Geometry check sheet. Reference: the model listing, model coordinates, mm. A direction names the side the tool comes from. Round coordinates to 2 decimals unless told otherwise and drop trailing zeros. Write each loop counter-clockwise with the first axis right and the second up, starting at its lowest first coordinate (ties: lowest second). Pieces come first, ordered by that corner, then holes.
from build123d import *

# Parameters (mm, degrees)
BOSS_EXTRUDE1_DEPTH = 15.3
SHELL1_T            = 3
SKETCH2_W           = 7
SKETCH2_H           = 15.5
SKETCH2_W_2         = 3
SKETCH2_W_3         = 15.5
SKETCH2_H_2         = 7
SKETCH2_H_3         = 3
CUT_EXTRUDE1_DEPTH  = 5


with BuildPart() as part:
    # Sketch1 → Boss-Extrude1 (new body)
    with BuildSketch(Plane.XY):
        Polygon((0, 0), (15.5, 0), (15.5, 30), (45.5, 30), (45.5, 45.5), (0, 45.5), align=None)
    extrude(amount=BOSS_EXTRUDE1_DEPTH)

    # Shell1
    shell1_openings = [part.faces().sort_by_distance(p)[0] for p in [
        (7.75, 0, 7.65),
        (45.5, 37.75, 7.65),
    ]]
    offset(amount=SHELL1_T, openings=shell1_openings, kind=Kind.INTERSECTION)

    # Sketch2 → Cut-Extrude1 (cut)
    with BuildSketch(Plane.XY.offset(18.3)):
        Polygon((15.5, 30), (16.5, 30), (16.5, 45.5), (0, 45.5), (0, 29), (15.5, 29), align=None)
        with Locations((23, 37.75)):
            Rectangle(SKETCH2_W, SKETCH2_H)
        with Locations((33, 37.75)):
            Rectangle(SKETCH2_W, SKETCH2_H)
        with Locations((41, 37.75)):
            Rectangle(SKETCH2_W_2, SKETCH2_H)
        with Locations((7.75, 22.5)):
            Rectangle(SKETCH2_W_3, SKETCH2_H_2)
        with Locations((7.75, 12.5)):
            Rectangle(SKETCH2_W_3, SKETCH2_H_2)
        with Locations((7.75, 4.5)):
            Rectangle(SKETCH2_W_3, SKETCH2_H_3)
    extrude(amount=-CUT_EXTRUDE1_DEPTH, mode=Mode.SUBTRACT)


solid = part.part
1. Section check C-C (y = 34.5). Record the cut outline in (x, z), plus the area to 3 significant figures.
2. Release check for a two-part mould opening along Z. For faces 1 (the face through (18, 38, 15.3)), 2 (the face through (44, 38, 15.3)), 3 (the face through (16, 30, -3)), 4 (the face through (42.5, 38, 17)) record: +Z half, -Z half, draft (parallel to the pull), parting line (faces both ways), or undercut.
3. Section check B-B (x = 3.5). Record the cut outline in (y, z).
4. Depth check by flat-ended pin: pin 1 Ø6.5 at (y, z) = (9, 9) entering from +X; pin 2 Ø10.5 at (x, z) = (38.5, 11.5) entering from -Y. Enter the tip coordinate at first touch or a pass-through.
5. Section check A-A (z = 4). Record the cut outline in (x, y).
6. Scan lines: line 1 along X through (y, z) = (31, 17.25); line 2 along Y through (x, z) = (11, 15.5); line 3 along X through (y, z) = (22, 1.75). Record each from-to range of solid material in increasing order.
7. Access from +Z, -Z, +X, -X, +Y, -Y to the whole of each face (thin tool, end or side, straight path). Record for faces 5 (the face through (38, 38, 15.3)), 6 (the face through (8, 8, 15.3)), 7 (the face through (32, 27, 8)), 8 (the face through (45.5, 38, 17)), 9 (the face through (8, 29, 17)).
8. Section check D-D (x = 28). Record the cut outline in (y, z).
Results below:
1. outline: (-3, -3) - (45.5, -3) - (45.5, 0) - (0, 0) - (0, 18.3) - (-3, 18.3) - close; (16.5, 15.3) - (19.5, 15.3) - (19.5, 18.3) - (16.5, 18.3) - close; (26.5, 15.3) - (29.5, 15.3) - (29.5, 18.3) - (26.5, 18.3) - close; (36.5, 15.3) - (39.5, 15.3) - (39.5, 18.3) - (36.5, 18.3) - close; (42.5, 15.3) - (45.5, 15.3) - (45.5, 18.3) - (42.5, 18.3) - close
1. area: 236 mm2
2. face 1: undercut
2. face 2: undercut
2. face 3: -Z half
2. face 4: draft
3. outline: (0, -3) - (48.5, -3) - (48.5, 18.3) - (45.5, 18.3) - (45.5, 0) - (0, 0) - close; (0, 15.3) - (3, 15.3) - (3, 18.3) - (0, 18.3) - close; (6, 15.3) - (9, 15.3) - (9, 18.3) - (6, 18.3) - close; (16, 15.3) - (19, 15.3) - (19, 18.3) - (16, 18.3) - close; (26, 15.3) - (29, 15.3) - (29, 18.3) - (26, 18.3) - close
4. pin 1: stops at x = 18.5
4. pin 2: stops at y = 27
5. outline: (-3, 0) - (0, 0) - (0, 45.5) - (45.5, 45.5) - (45.5, 48.5) - (-3, 48.5) - close; (15.5, 0) - (18.5, 0) - (18.5, 27) - (45.5, 27) - (45.5, 30) - (15.5, 30) - close
6. line 1: x = -3 to 0, 16.5 to 19.5, 26.5 to 29.5, 36.5 to 39.5, 42.5 to 45.5
6. line 2: y = 0 to 3, 6 to 9, 16 to 19, 26 to 29, 45.5 to 48.5
6. line 3: x = -3 to 0, 15.5 to 18.5
7. face 5: +X
7. face 6: -Y
7. face 7: +Z, -Z, +X, -Y
7. face 8: +Z, -Z, +X, +Y, -Y
7. face 9: +Z
8. outline: (27, -3) - (48.5, -3) - (48.5, 18.3) - (27, 18.3) - close; hole (30, 0) - (45.5, 0) - (45.5, 15.3) - (30, 15.3) - close
